The figure shows three views and two pictorial views of one solid part (mm, origin at its lowest corner). Answer the questions. Round coordinates to 2 decimals unless told otherwise and drop trailing zeros. Order: outer loops, then holes, each group sorted by start corner. A loop starts at its lowest first (then second) coordinate and runs counter-clockwise, first axis right, second up. Notation, with made-up numbers: M 32,66.5 L 40,66.5 A9 ccw 40,80.5 Z; hole C 49.25,68 d2. An arc over 180 degrees is marked long. Return JSON: item names as keys, results as strings.
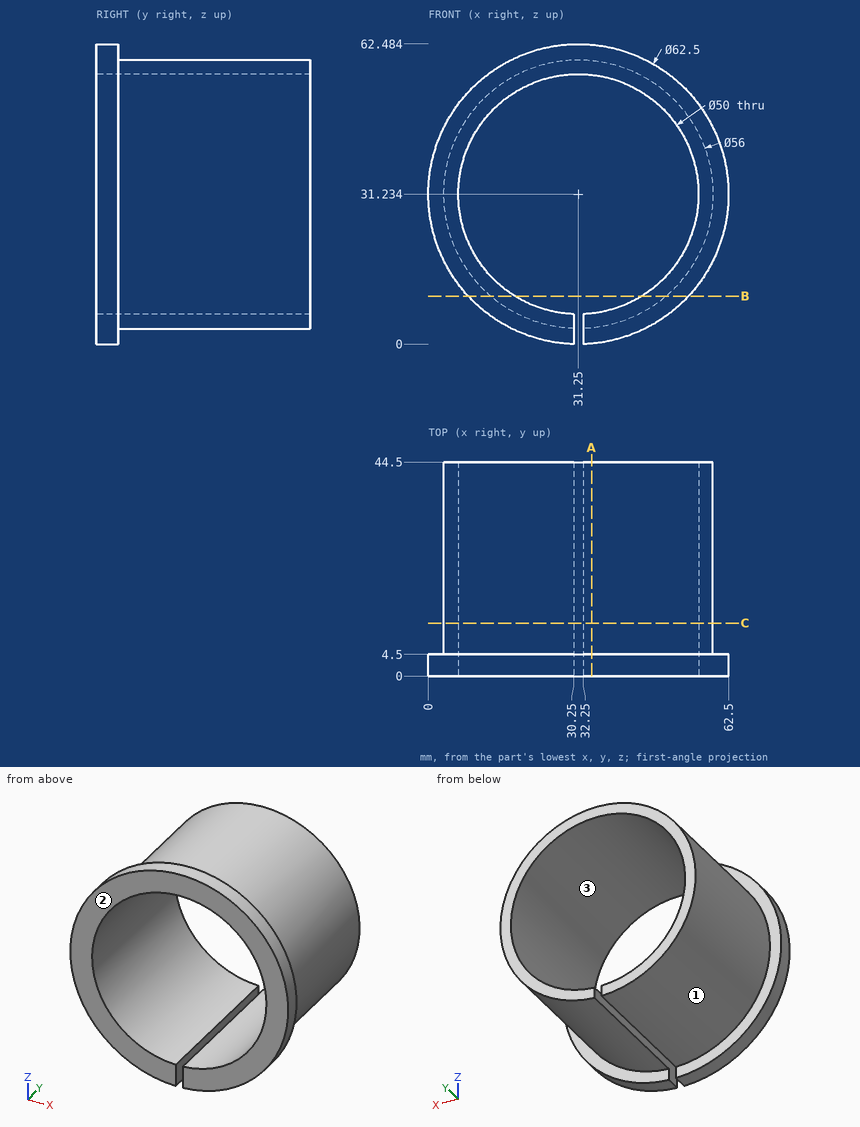
Item 1: Each of these flat-tipped pins is pushed along its axis until it touches: pin 1 (5 mm diameter, centred on y = 35, z = 48.5, fed in from -X); pin 2 (3 mm diameter, centred on y = 23.5, z = 43.5, fed in from +X); pin 3 (10 mm diameter, centred on y = 37, z = 53, fed in from -X); pin 4 (2 mm diameter, centred on x = 49, z = 17.5, fed in from -Y). Where does it stop, or does it pass through?
Output:
{"pin 1": "stops at x = 7.46", "pin 2": "stops at x = 57.1", "pin 3": "stops at x = 8.82", "pin 4": "passes through"}
Item 2: The mould has two halves that part along Z. Classify the marked faces 1, 2 and 3: pulls with the +Z half, pulls with the -Z half, needs draft (parallel to the pull), parting line crosses it, or undercut.
Output:
{"face 1": "parting line crosses it", "face 2": "needs draft", "face 3": "undercut"}
Item 3: Find section B-B (z = 10). Determine the outline of the cut face in (x, y), plus the area to 3 significant figures.
Output:
{"outline": "M 8.32,0 L 18.05,0 L 18.05,44.5 L 13,44.5 L 13,4.5 L 8.32,4.5 Z; M 44.45,0 L 54.18,0 L 54.18,4.5 L 49.5,4.5 L 49.5,44.5 L 44.45,44.5 Z", "area": "492 mm^2"}
Item 4: Find section A-A (x = 34). Determine the outline of the cut face in (y, z).
Output:
{"outline": "M 0,0.11 L 4.5,0.11 L 4.5,3.37 L 44.5,3.37 L 44.5,6.39 L 0,6.39 Z; M 0,56.08 L 44.5,56.08 L 44.5,59.1 L 4.5,59.1 L 4.5,62.36 L 0,62.36 Z"}
Item 5: Consider line 1 along Y through (x, z) = (56, 17.5); line 2 along X through (y, z) = (25.5, 43.5); line 3 along Z through (x, y) = (53.5, 25.5) (3 decimals). Determine where each line is inside the solid, lowest interval first. Write a range as [from, to].
Output:
{"line 1": "y = [0, 4.5]", "line 2": "x = [6.08, 9.47], [53.03, 56.42]", "line 3": "z = [14.236, 19.835], [42.633, 48.232]"}
Item 6: Find section C-C (y = 11). Determine the outline of the cut face in (x, z).
Output:
{"outline": "M 30.25,3.25 L 30.25,6.25 A25 cw long 32.25,6.25 L 32.25,3.25 A28 ccw long Z"}
